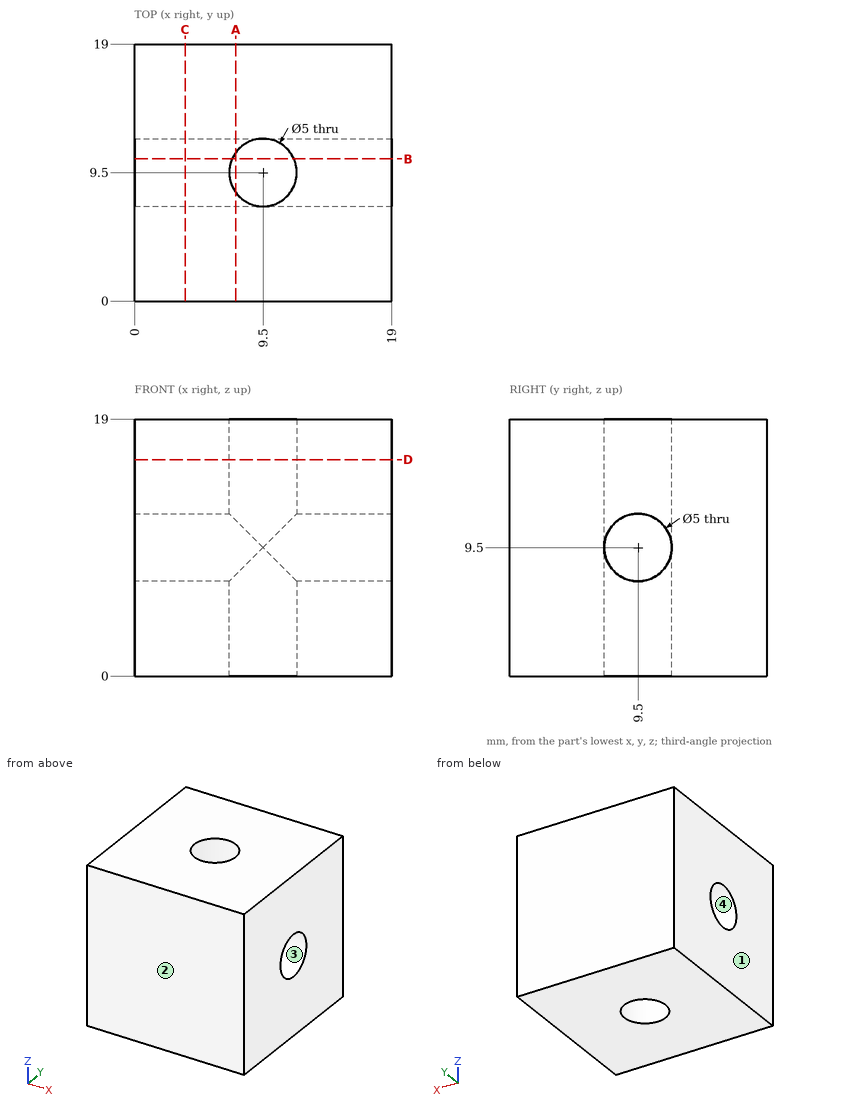
Here's the drawing with two shaded views (mm, measured from the low corner). I have some questions. Give positions to 0.01 mm unless a question says otherwise; leave off trailing zeros. Write each loop counter-clockwise with the first axis right and the second up, starting at its lowest first coordinate (ties: lowest second). Pieces come first, ordered by that corner, then holes. Notation, with made-up numbers: (0.5, 84) - (56.5, 84) arc R34 cw to (56.5, 117) - close; hole circle Ø3 at (-2, 17.25). An arc over 180 degrees is marked (long way). One line per item, written item: value. Start each with the question number.
Item 1: Imagine slicing it at C-C, the plane x = 3.75. List the corners of the cut face in (y, z) for me, and give its area (3 significant figures).
Item 2: Imagine slicing it at B-B, the plane y = 10.5. List the corners of the cut face in (x, z) for me.
Item 3: If we mould it in two halves opening along Y, with no side actions, what happens to the marked faces 1, 2, 3 and 4? For each: +Y half, -Y half, draft (parallel to the pull), parting line (faces both ways), or undercut.
Item 4: Imagine slicing it at A-A, the plane x = 7.5. List the corners of the cut face in (y, z) for me, and give its area (3 significant figures).
Item 5: Please list where this line runs through material, in increasing order: line 1 (Z direction, x = 13.5, y = 9.5). Write a range as from..to.
Item 6: I'm going to push a flat-ended pin straight in: pin 1 (4.5 mm diameter, centred on y = 9.5, z = 9.5, fed in from -X). Where does the tip first touch, or does it pass through?
Geometry says:
1. outline: (0, 0) - (19, 0) - (19, 19) - (0, 19) - close; hole circle Ø5 at (9.5, 9.5)
1. area: 341 mm^2
2. outline: (0, 0) - (7.21, 0) - (7.21, 7.21) - (0, 7.21) - close; (0, 11.79) - (7.21, 11.79) - (7.21, 19) - (0, 19) - close; (11.79, 0) - (19, 0) - (19, 7.21) - (11.79, 7.21) - close; (11.79, 11.79) - (19, 11.79) - (19, 19) - (11.79, 19) - close
3. face 1: draft
3. face 2: -Y half
3. face 3: undercut
3. face 4: undercut
4. outline: (0, 0) - (8, 0) - (8, 7.5) arc R2.5 cw to (8, 11.5) - (8, 19) - (0, 19) - close; (11, 0) - (19, 0) - (19, 19) - (11, 19) - (11, 11.5) arc R2.5 cw to (11, 7.5) - close
4. area: 298 mm^2
5. line 1: 0..7, 12..19
6. pin 1: through
